```python
from build123d import *

# Parameters (mm, degrees)
F3_DEPTH = 20
F4_W     = 1.2972189062
F4_H     = 10.2779610492
F6_W     = 7
F6_H     = 12
F7_DEPTH = 37.6
F8_R     = 5
F9_DEPTH = 44.8


with BuildPart() as f1:
    # F0 (on Front) → F1 (revolve)
    with BuildSketch(Plane.XZ):
        with BuildLine():
            add(Edge.make_bspline(
                [(0, 30), (16.2610174256, 30), (25, 10.9921857571), (25, 0)],
                knots=[0, 0, 0, 0, 39.0512483795, 39.0512483795, 39.0512483795, 39.0512483795], degree=3))
            add(Edge.make_bspline(
                [(0, 30), (-9.0857928701, 30), (-15.8232208718, 24.065796812), (-20, 16.9113518854)],
                knots=[0, 0, 0, 0, 21.8197634754, 21.8197634754, 21.8197634754, 21.8197634754], degree=3))
            Line((-20, 16.9113518854), (-20, 0))
            Line((-20, 0), (25, 0))
        make_face()
    revolve(axis=Axis((12.5, 0, 0), (1, 0, 0)))

    # F2 (on Front) → F3 (cut, symmetric)
    with BuildSketch(Plane.XZ):
        Polygon((26.4112874866, 18.832474947), (19.5291824639, 19.1946905106), (19.5291824639, 7.9659949988), (26.4112874866, 4.5249424875), align=None)
        Polygon((19.5291824639, -7.9659949988), (19.5291824639, -19.1946905106), (26.4112874866, -18.832474947), (26.4112874866, -4.5249424875), align=None)
    extrude(amount=F3_DEPTH, both=True, mode=Mode.SUBTRACT)

    # F4 (on Front) → F5 (revolve, cut)
    with BuildSketch(Plane.XZ):
        with Locations((14.3513905469, 26.2715257704)):
            Rectangle(F4_W, F4_H)
    revolve(axis=Axis((7.8121407423, 0, 0), (1, 0, 0)), mode=Mode.SUBTRACT)

    # F6 (on Front) → F7 (join)
    with BuildSketch(Plane.XZ):
        with Locations((-7.5, 0)):
            Rectangle(F6_W, F6_H)
    extrude(amount=F7_DEPTH)

    # F8 (on Front) → F9 (join)
    with BuildSketch(Plane.XZ):
        with Locations((-7.6043987647, 0)):
            Circle(F8_R)
    extrude(amount=-F9_DEPTH)


solid = f1.part
```
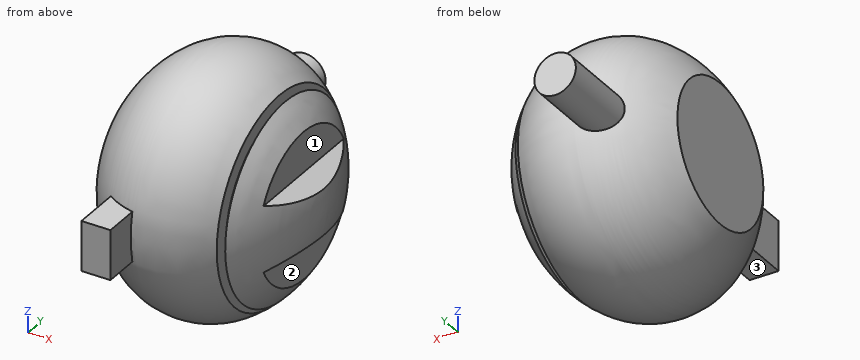
Source: CAD feature listing. Evaluate the final solid. Frame: model axes, mm. Face numbers are marked on the shaded views. A direction names the side the tool comes from. Coordinates: 2 decimals unless noted, no trailing zeros. Use a Markdown table: item, result. Add a question column.
Q1. Access query for the marked faces 1, 2 and 3. Directions: +Z, -Z, +X, -X, +Y, -Y. A direction counts if a zero-diameter tool reaches every point of the face in a straight line with its end or side. Return the directions, or none.
Q2. Material intervals for L1, parallel to Y at x = -16, z = 7.5; L2, parallel to X at y = -1.5, z = 14; L3, parallel to Y at x = 8, z = -13.5, sorted ascending.
Q3. First-contact query: pin 1 (10 mm diameter, centred on x = -1, z = -21.5, fed in from -Y); pin 2 (2 mm diameter, centred on y = 4.5, z = -20.5, fed in from -X); pin 3 (5 mm diameter, centred on y = 0, z = -13.5, fed in from +X); pin 4 (3 mm diameter, centred on x = 12.5, y = -28, fed in from -Z). Flat tips, straight axial feed; report the tip coordinate or a pass-through.
Result:
| question | item | result |
|---|---|---|
| 1 | face 1 | +Z, +X, +Y, -Y |
| 1 | face 2 | -Z, +X, +Y, -Y |
| 1 | face 3 | -Z, -X, -Y |
| 2 | L1 | y = -21.12 to 21.12 |
| 2 | L2 | x = -20 to 19.53 |
| 2 | L3 | y = -24.91 to 24.91 |
| 3 | pin 1 | stops at y = -25.03 |
| 3 | pin 2 | stops at x = -17.98 |
| 3 | pin 3 | stops at x = 19.53 |
| 3 | pin 4 | passes through |
